Check sheet for the modelled part. Datum: model origin and axes. Units: mm. Face numbers are marked on the shaded views. A direction names the side the tool comes from. Give positions to 0.01 mm unless a question says otherwise; leave off trailing zeros. Loops run counter-clockwise (first coordinate to the right, second up) from the corner with the lowest first, then second, coordinate; pieces in that order, holes last. Notation, with made-up numbers: (26, 49) -> (68, 49) arc R19 ccw to (68, 69) -> close; hole circle Ø7 at (56, -23). An arc over 180 degrees is marked (long way). Write each question's results on one line, items separated by ' | '. Start each with the question number.
Item 1: Cross-section at B-B on z = 58. Enter the section's corners in (x, y).
Item 2: Gauge pin test, flat ends, axial feed: pin 1 Ø1 at (y, z) = (-69, 97.5) entering from +X; pin 2 Ø1.5 at (y, z) = (-31.5, 114) entering from -X; pin 3 Ø3 at (x, y) = (43.5, 70) entering from +Z. Record the tip position at first contact, or that the pin passes through.
Item 3: Cross-section at C-C on y = 65.5. Enter the section's corners in (x, z), then the cut area to 3 significant figures.
Item 4: Scan lines: line 1 along X through (y, z) = (12, 76); line 2 along Y through (x, z) = (51.5, 148.5); line 3 along Z through (x, y) = (-1, 52). Record each from-to range of solid material in increasing order.
Item 5: Mould release check, pull along X, two halves, no side actions. Record for the marked faces 1, 2 and 3: pulls with the +X half, pulls with the -X half, needs draft (parallel to the pull), parting line crosses it, or undercut.
Item 6: Access from +Z, -Z, +X, -X, +Y, -Y to the whole of each face (thin tool, end or side, straight path). Record for the marked faces 4, 5, 6 and 7.
Item 7: Cross-section at A-A on x = 79.5. Enter the section's corners in (y, z), then the cut area to 3 significant figures.
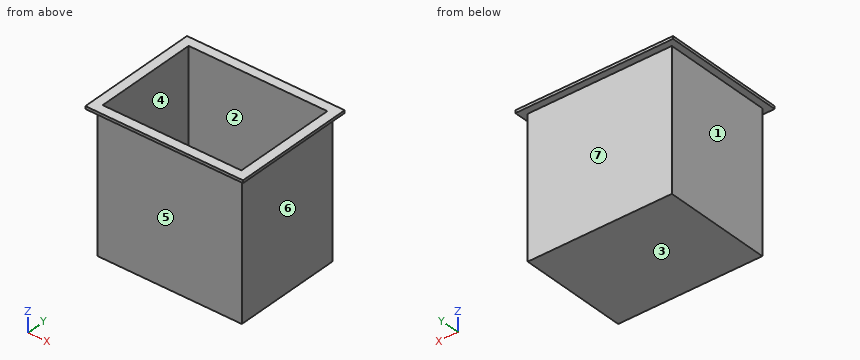
from build123d import *

# Parameters (mm, degrees)
SKETCH_W      = 204.8
SKETCH_H      = 153.6
PAD_DEPTH     = 204.8
THICKNESS_T   = 4
SKETCH001_W   = 232.8
SKETCH001_H   = 181.6
SKETCH001_W_2 = 212.8
SKETCH001_H_2 = 161.6
PAD001_DEPTH  = 4


with BuildPart() as part:
    # Sketch → Pad (new body)
    with BuildSketch(Plane.XY):
        Rectangle(SKETCH_W, SKETCH_H)
    extrude(amount=PAD_DEPTH)

    # Thickness
    thickness_openings = [part.faces().sort_by_distance(p)[0] for p in [
        (0, 0, 204.8),
    ]]
    offset(amount=THICKNESS_T, openings=thickness_openings, kind=Kind.INTERSECTION)

    # Sketch001 → Pad001 (new body)
    with BuildSketch(Plane.XY.offset(204.8)):
        Rectangle(SKETCH001_W, SKETCH001_H)
        Rectangle(SKETCH001_W_2, SKETCH001_H_2, mode=Mode.SUBTRACT)
    extrude(amount=-PAD001_DEPTH)


solid = part.part
Answer sheet:
1) outline: (-106.4, -80.8) -> (106.4, -80.8) -> (106.4, 80.8) -> (-106.4, 80.8) -> close; hole (-102.4, -76.8) -> (102.4, -76.8) -> (102.4, 76.8) -> (-102.4, 76.8) -> close
2) pin 1: stops at x = 106.4 | pin 2: stops at x = -106.4 | pin 3: stops at z = 0
3) outline: (-116.4, 200.8) -> (-106.4, 200.8) -> (-106.4, -4) -> (106.4, -4) -> (106.4, 200.8) -> (116.4, 200.8) -> (116.4, 204.8) -> (102.4, 204.8) -> (102.4, 0) -> (-102.4, 0) -> (-102.4, 204.8) -> (-116.4, 204.8) -> close | area: 2,570 mm²
4) line 1: x = -106.4 to -102.4, 102.4 to 106.4 | line 2: y = -80.8 to -76.8, 76.8 to 80.8 | line 3: z = -4 to 0
5) face 1: pulls with the -X half | face 2: undercut | face 3: needs draft
6) face 4: +Z | face 5: -Z, +X, -X, -Y | face 6: -Z, +X, +Y, -Y | face 7: -Z, +X, -X, +Y
7) outline: (-90.8, 200.8) -> (-80.8, 200.8) -> (-80.8, -4) -> (80.8, -4) -> (80.8, 200.8) -> (90.8, 200.8) -> (90.8, 204.8) -> (76.8, 204.8) -> (76.8, 0) -> (-76.8, 0) -> (-76.8, 204.8) -> (-90.8, 204.8) -> close | area: 2,360 mm²
